Can you work these out from the model? Positions are in its coordinate system, mm. Face numbers are marked on the shaded views. A direction names the side the tool comes from. Give positions to 0.01 mm unless a question says otherwise; leave off trailing zeros. Loops run counter-clockwise (first coordinate to the right, second up) from the corner with the lowest first, then second, coordinate; pieces in that order, holes last. Notation, with made-up numbers: M 65.5,41 L 93.5,41 A18 ccw 93.5,46 Z; hole C -11.75,16.5 d5. An arc over 180 degrees is marked long. Use CSV: the item, a comma, the result in double quotes.
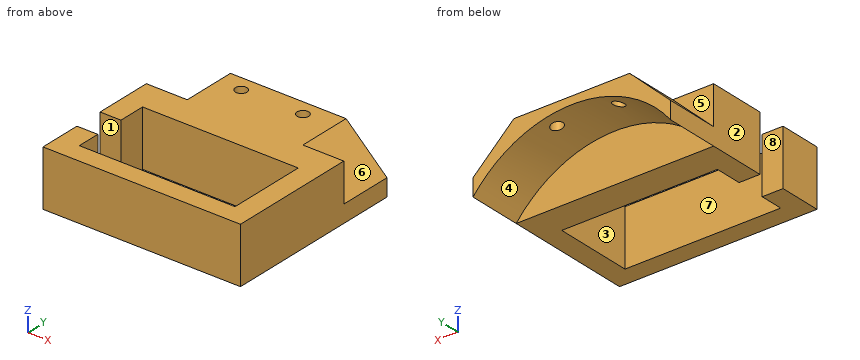
Autodesk Inventor part; units mm, degrees
ref_plane "YZ Plane" through (0, 0, 0) normal (1, 0, 0) x (0, 1, 0)
ref_plane "XZ Plane" through (0, 0, 0) normal (0, 1, 0) x (-1, 0, 0)
ref_plane "XY Plane" through (0, 0, 0) normal (0, 0, 1) x (1, 0, 0)
ref_plane "Plano de trabajo1" through (16, 0, 22.5) normal (0, 0, -1) x (-1, 0, 0)
sketch "Boceto2" plane through (16, 0, 22.5) normal (0, 0, -1) x (-1, 0, 0)
  line L0 (-6.5, 0) -> (0, 0)
  line L1 (0, 0) -> (32, 0)
  circle A0 centre (8, 8) radius 1.5
  circle A1 centre (24, 8) radius 1.5
  point P0 (16, 0)
  dimension "d15" = 3
  dimension "d16" = 3
extrude "Extrusión2" [suppressed]
ref_plane "Plano de trabajo2" through (0, 0, 0) normal (0, -1, 0) x (1, 0, 0)
sketch "Boceto4" plane through (0, 0, 0) normal (0, -1, 0) x (1, 0, 0)
  circle A0 centre (0, 0) radius 32.5
  arc A1 (28.2887, 16) -> (-28.2887, 16) centre (0, 0) ccw
  line L0 (0, 32.5) -> (0, 34.5)
  line L1 (0, 34.5) -> (-26.2329, 34.5)
  line L2 (-26.2329, 34.5) -> (30.7149, 34.5)
  line L3 (0, 0) -> (0, 20)
  arc A2 (28.2887, 16) -> (-28.2887, 16) centre (0, 0) ccw
  line L4 (0, 20) -> (50, 20)
  line L5 (50, 20) -> (-50, 20)
  line L6 (0, 34.5) -> (15, 34.5)
  line L7 (15, 34.5) -> (25.6174, 20)
  line L8 (0, 34.5) -> (-15, 34.5)
  line L9 (-15, 34.5) -> (-25.6174, 20)
  point P0 (-25.6174, 20)
  dimension "d19" = 2
  dimension "d20" = 20
  dimension "d21" = 50
  dimension "d22" = 100
  dimension "d23" = 15
  dimension "d24" = 15
extrude "Extrusión3" add sketch "Boceto4" against normal blind 12 contours A0 L0 L2 L7 | L9 L1 L0 A0
sketch "Boceto5" plane through (-15, 0, 34.5) normal (0, 0, 1) x (1, 0, 0)
  line L0 (30, 0) -> (30, 12)
  line L1 (30, 0) -> (30, 8)
  line L2 (30, 8) -> (22, 8)
  line L3 (22, 8) -> (6, 8)
  circle A0 centre (22, 8) radius 1.5
  circle A1 centre (6, 8) radius 1.5
  point P0 (15, 0)
  dimension "d27" = 8
  dimension "d28" = 8
  dimension "d29" = 16
  dimension "d30" = 3
  dimension "d31" = 3
extrude "Extrusión4" cut sketch "Boceto5" against normal blind 12
sketch "Boceto6" plane through (0, 0, 0) normal (0, -1, 0) x (1, 0, 0)
  circle A0 centre (0, 0) radius 32.5
  arc A1 (25.6174, 20) -> (-25.6174, 20) centre (0, 0) ccw
  line L0 (-15, 34.5) -> (15, 34.5)
  line L1 (25.6174, 20) -> (15, 34.5)
  line L2 (15, 34.5) -> (-15, 34.5)
  line L3 (-15, 34.5) -> (-25.6174, 20)
extrude "Extrusión5" add sketch "Boceto6" along normal blind 2 contours A0 L3 L0 L1
sketch "Boceto7" plane through (0, -2, 0) normal (0, -1, 0) x (1, 0, 0)
  line L0 (-25.6174, 20) -> (-15, 34.5)
  line L1 (-15, 34.5) -> (-25.6174, 34.5)
  line L2 (-25.6174, 34.5) -> (-25.6174, 20)
  line L3 (-25.6174, 20) -> (25.6174, 20)
  line L4 (25.6174, 20) -> (25.6174, 34.5)
  line L5 (25.6174, 20) -> (15, 34.5)
  line L6 (15, 34.5) -> (25.6174, 34.5)
  circle A0 centre (0, 0) radius 32.5
  line L7 (-15, 34.5) -> (15, 34.5)
extrude "Extrusión6" add sketch "Boceto7" along normal blind 8 contours L2 L1 L0 | A0 L3 | L0 L7 L5 A0 | L5 L6 L4 picked at (-1.7193, 25.9173)
sketch "Boceto8" plane through (-15, 12, 34.5) normal (0, 0, 1) x (1, 0, 0)
  line L0 (40.6174, -22) -> (-10.6174, -22)
  line L1 (-10.6174, -22) -> (-10.6174, -42.5)
  line L2 (-10.6174, -42.5) -> (39.7361, -42.5)
  line L3 (40.6174, -22) -> (40.6174, -42.5)
  line L4 (40.6174, -42.5) -> (39.7361, -42.5)
  line L5 (-10.6174, -22) -> (40.6174, -22)
  line L6 (40.6174, -14) -> (40.6174, -22)
  line L7 (-10.6174, -22) -> (40.6174, -22)
  line L8 (15, -22) -> (35.2, -22)
  line L9 (35.2, -22) -> (35.2, -42.5)
  line L10 (15, -22) -> (-5.2, -22)
  line L11 (-5.2, -22) -> (-5.2, -42.5)
  line L12 (-5.2, -42.5) -> (-5.2, -37.5)
  line L13 (-5.2, -22) -> (-5.2, -29)
  line L14 (-5.2, -29) -> (-10.6174, -29)
  line L15 (-5.2, -42.5) -> (-5.2, -36.5)
  line L16 (-5.2, -36.5) -> (-10.6174, -36.5)
  point P0 (15, -12)
  dimension "d38" = 20.5
  dimension "d39" = 20.5
  dimension "d40" = 20.2
  dimension "d41" = 20.2
  dimension "d43" = 7
  dimension "d44" = 6
extrude "Extrusión7" add sketch "Boceto8" against normal blind 14.5 contours L3 L4 L2 L9 L0 | L11 L14 L1 L0 | L2 L1 L16 L11
sketch "Boceto9" plane through (20.2, -30.5, 34.5) normal (0, -1, 0) x (1, 0, 0)
  line L0 (5.4174, -14.5) -> (5.4174, 0)
  line L1 (-45.8174, 0) -> (-45.8174, -14.5)
  line L2 (5.4174, 0) -> (-45.8174, 0)
  line L3 (-45.8174, 0) -> (-45.8174, -14.5)
  line L4 (-45.8174, -14.5) -> (5.4174, -14.5)
  line L5 (5.4174, 0) -> (-5.2, 0)
  line L6 (5.4174, -14.5) -> (5.4174, 0)
  point P0 (-20.2, -34.5)
extrude "Extrusión8" add sketch "Boceto9" along normal blind 5
sketch "Boceto10" plane through (0, -2, 0) normal (0, 1, 0) x (1, 0, 0)
  line L0 (-15, -34.5) -> (-25.6174, -34.5)
  line L1 (-15, -34.5) -> (-25.6174, -34.5)
  line L2 (-25.6174, -34.5) -> (-25.6174, -24.5)
  line L3 (-25.6174, -34.5) -> (-25.6174, -20)
  line L4 (-25.6174, -24.5) -> (-15, -34.5)
  line L5 (-25.6174, -20) -> (25.6174, -20)
  line L6 (-25.6174, -24.5) -> (-25.6174, -20)
  line L7 (-25.6174, -20) -> (-15, -34.5)
  line L8 (-15, -34.5) -> (-25.6174, -20)
  arc A0 (-25.6174, -20) -> (25.6174, -20) centre (0, 0) ccw
  line L9 (0, -32.5) -> (0, -25.3096)
  line L10 (15, -34.5) -> (25.6174, -34.5)
  line L11 (25.6174, -34.5) -> (25.6174, -24.5)
  line L12 (25.6174, -34.5) -> (25.6174, -20)
  line L13 (25.6174, -24.5) -> (15, -34.5)
  line L14 (25.6174, -20) -> (15, -34.5)
  dimension "d49" = 10
extrude "Extrusión9" add sketch "Boceto10" along normal blind 14 contours L12 L13 L14 | L4 L3 L7
sketch "Boceto11" plane through (-25.6174, -17, 34.5) normal (0, 0, 1) x (1, 0, 0)
  line L0 (45.8174, 7) -> (45.8174, -13.5)
  line L1 (45.8174, -13.5) -> (45.8174, 7)
  line L2 (45.8174, 7) -> (45.8174, -3.25)
  point P0 (25.6174, 17)
properties part number "brazo_articulado_2"
Q1. I'm going to push flat-ended pins straight in: P1, Ø6, axis at x = -23, z = 27, coming from the +Y side; P2, Ø10, axis at x = 0.5, y = 4.5, coming from the -Z side; P3, Ø2.5, axis at x = -9, y = 8, coming from the +Z side; P4, Ø5, axis at x = 1.5, z = 27, coming from the +Y side. Where does each tip first touch, or does it pass through?
Model answer:
P1,"y = 12"
P2,"z = 32.03"
P3,"through"
P4,"y = -2"
Q2. For the marked faces 1, 2, 3, 4 and 5, which set-ups out of +Z, -Z, +X, -X, +Y, -Y let a thin tool reach every point of the face, with its end or its side?
Model answer:
face 1,"+Z, -Z, -X"
face 2,"+Z, -Z, -X, +Y, -Y"
face 3,"+Z, -Z"
face 4,"-Z, +Y"
face 5,"+Z, -X, +Y"
Q3. I want a section at B-B, the plane y = 8. Please give me the cut outline in (x, z), then the cut area to 3 significant figures.
Model answer:
outline,"M -25.62,20 A32.5 cw -10.5,30.76 L -10.5,34.5 L -15,34.5 L -25.62,24.5 Z; M -7.5,31.62 A32.5 cw 5.5,32.03 L 5.5,34.5 L -7.5,34.5 Z; M 8.5,31.37 A32.5 cw 25.62,20 L 25.62,24.5 L 15,34.5 L 8.5,34.5 Z"
area,"172 mm2"
Q4. If we mould it in two halves opening along X, with no side actions, what happens to the marked faces 6, 7 and 8? For each: released by +X, released by -X, zero draft, split by the parting line, or undercut.
Model answer:
face 6,"released by +X"
face 7,"undercut"
face 8,"zero draft"
Q5. I want a section at C-C, the plane x = 7. Please give me the cut outline in (y, z).
Model answer:
outline,"M -35.5,20 L -30.5,20 L -30.5,34.5 L -35.5,34.5 Z; M -10,20 L -2,20 L -2,31.74 L 6.5,31.74 L 6.5,34.5 L -10,34.5 Z; M 9.5,31.74 L 12,31.74 L 12,34.5 L 9.5,34.5 Z"
Q6. I want a section at D-D, the plane z = 33.5. Please give me the cut outline in (x, y), then the cut area to 3 significant figures.
Model answer:
outline,"M -25.62,-35.5 L 25.62,-35.5 L 25.62,-2 L 16.06,-2 L 16.06,12 L -16.06,12 L -16.06,-2 L -25.62,-2 L -25.62,-17 L -20.2,-17 L -20.2,-10 L 20.2,-10 L 20.2,-30.5 L -20.2,-30.5 L -20.2,-24.5 L -25.62,-24.5 Z; hole C -9,8 d3; hole C 7,8 d3"
area,"1,280 mm2"
Q7. I want a section at A-A, the plane y = -14. Please give me the cut outline in (x, z), then the cut area to 3 significant figures.
Model answer:
outline,"M -25.62,20 L -20.2,20 L -20.2,34.5 L -25.62,34.5 Z; M 20.2,20 L 25.62,20 L 25.62,34.5 L 20.2,34.5 Z"
area,"157 mm2"
Q8. Please list where these lines run through material, in increasing order: L1, parallel to Y at x = 7, z = 33.6; L2, parallel to Y at x = -19.5, z = 23.5; L3, parallel to X at y = 8, z = 33.3. Write a range as from..to.
Model answer:
L1,"-35.5..-30.5, -10..6.5, 9.5..12"
L2,"-35.5..-30.5, -10..-2"
L3,"-16.27..-10.5, -7.5..5.5, 8.5..16.27"
